Can you work these out from the model? Positions are in its coordinate system, mm. Face numbers are marked on the shaded views. A direction names the side the tool comes from. Coordinates: 2 decimals unless noted, no trailing zeros. Order: outer loops, then holes, each group sorted by start corner. A loop starts at its lowest first (then second) coordinate and runs counter-clockwise, first axis right, second up. Notation, with made-up numbers: (59.5, 45) -> (78.5, 45) arc R34 cw to (78.5, 77) -> close; hole circle Ø7 at (-32.5, 84). An arc over 180 degrees is marked (long way). Answer as a JSON object with one key per item and string values. Group by question number.
(1) I want a section at B-B, the plane y = 11.7. State how many separate pieces and enclosed holes the cut face has, plus the area to 3 significant figures.
(2) For pin 1 (1.2 mm diameter, centred on x = 8, y = 37, fed in from -Z); pin 2 (4 mm diameter, centred on x = 82.5, z = -12.5, fed in from -Y); pin 3 (0.8 mm diameter, centred on x = 130, y = 28.5, fed in from -Z), each with a flat end and sliding along its axis, tell me the tip position at first contact or that it passes through.
(3) I want a section at D-D, the plane y = 24. List the corners of the cut face in (x, z) for me, plus the area to 3 significant figures.
(4) I want a section at A-A, the plane z = -23. List the corners of the cut face in (x, y) for me, plus the area to 3 significant figures.
(5) I need wall thicknesses on line 1 (Y direction, x = 7.25, z = -13.25); line 2 (X direction, y = 37, z = -5); line 3 (Y direction, x = 129.75, z = -21). Which ranges of each line are inside material? Lowest first, please.
(6) If we mould it in two halves opening along X, with no side actions, what happens to the marked faces 3, 4, 5 and 6? For each: pulls with the +X half, pulls with the -X half, needs draft (parallel to the pull), parting line crosses it, or undercut.
(7) Which directions (+Z, -Z, +X, -X, +Y, -Y) give clear straight access to the entire face, cutting with the end or side of a thin tool? Please do the marked faces 1 and 2.
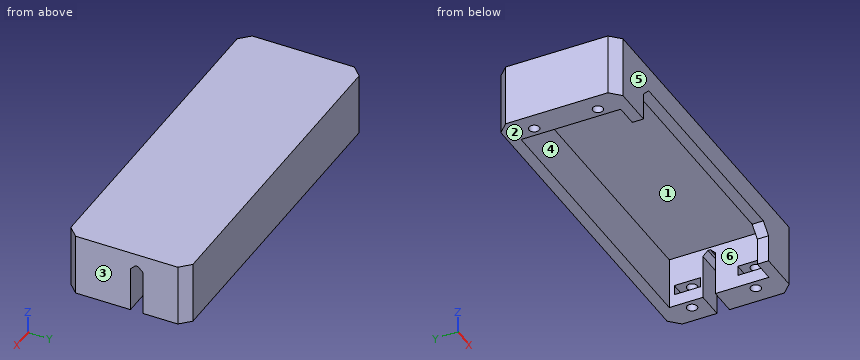
from build123d import *

# Parameters (mm, degrees)
SKETCH_W        = 137
SKETCH_H        = 49
SKETCH_R        = 2.05
SKETCH_W_2      = 115
SKETCH_H_2      = 40
PAD_DEPTH       = 25
CHAMFER_SIZE    = 4
SKETCH004_W     = 129
SKETCH004_H     = 41
PAD001_DEPTH    = 4
SKETCH003_W     = 7.55
SKETCH003_H     = 10.5
POCKET_DEPTH    = 4
POCKET001_DEPTH = 5.01
SKETCH005_W     = 22.132821
SKETCH005_H     = 5
POCKET002_DEPTH = 15
CHAMFER001_SIZE = 2


with BuildPart() as part:
    # Sketch → Pad (new body)
    with BuildSketch(Plane.XY):
        with Locations((68.5, 24.5)):
            Rectangle(SKETCH_W, SKETCH_H)
        with Locations((7.25, 11.7)):
            Circle(SKETCH_R, mode=Mode.SUBTRACT)
        with Locations((129.75, 11.7)):
            Circle(SKETCH_R, mode=Mode.SUBTRACT)
        with Locations((7.25, 37.3)):
            Circle(SKETCH_R, mode=Mode.SUBTRACT)
        with Locations((129.75, 37.3)):
            Circle(SKETCH_R, mode=Mode.SUBTRACT)
        with Locations((68.5, 24.5)):
            Rectangle(SKETCH_W_2, SKETCH_H_2, mode=Mode.SUBTRACT)
    extrude(amount=-PAD_DEPTH)

    # Chamfer
    chamfer_edges = [part.edges().sort_by_distance(p)[0] for p in [
        (137, 49, -12.5),
        (137, 0, -12.5),
        (0, 49, -12.5),
        (0, 0, -12.5),
    ]]
    chamfer(chamfer_edges, length=CHAMFER_SIZE)

    # Sketch004 → Pad001 (join)
    with BuildSketch(Plane.XY):
        with Locations((68.5, 24.5)):
            Rectangle(SKETCH004_W, SKETCH004_H)
    extrude(amount=-PAD001_DEPTH)

    # Sketch003 (on DatumPlane) → Pocket (cut)
    with BuildSketch(Plane.XY.offset(-20)):
        with Locations((7.25, 11.75)):
            Rectangle(SKETCH003_W, SKETCH003_H)
        with Locations((7.25, 37.25)):
            Rectangle(SKETCH003_W, SKETCH003_H)
        with Locations((129.75, 37.25)):
            Rectangle(SKETCH003_W, SKETCH003_H)
        with Locations((129.75, 11.75)):
            Rectangle(SKETCH003_W, SKETCH003_H)
    extrude(amount=POCKET_DEPTH, mode=Mode.SUBTRACT)

    # Sketch002 → Pocket001 (cut)
    with BuildSketch(Plane.XZ):
        Polygon((113, -10), (24, -10), (20, -14), (20, -147.795874), (117, -147.795874), (117, -14), align=None)
    extrude(amount=-POCKET001_DEPTH, mode=Mode.SUBTRACT)

    # Sketch005 (on DatumPlane) → Pocket002 (cut, symmetric)
    with BuildSketch(Plane.XY.offset(-20)):
        with Locations((131.19064, 28.5)):
            Rectangle(SKETCH005_W, SKETCH005_H)
    extrude(amount=POCKET002_DEPTH, both=True, mode=Mode.SUBTRACT)

    # Chamfer001
    chamfer001_edges = [part.edges().sort_by_distance(p)[0] for p in [
        (131.5, 26, -5),
        (131.5, 31, -5),
    ]]
    chamfer(chamfer001_edges, length=CHAMFER001_SIZE)


solid = part.part
Computed values:
{
 "1": {"separate pieces": "3", "enclosed holes": "0", "area": "810 mm2"},
 "2": {"pin 1": "stops at z = -4", "pin 2": "stops at y = 44.5", "pin 3": "stops at z = -5"},
 "3": {"outline": "(0, -25) -> (11, -25) -> (11, -4) -> (126, -4) -> (126, -25) -> (137, -25) -> (137, 0) -> (0, 0) -> close", "area": "1,010 mm2"},
 "4": {"outline": "(0, 4) -> (4, 0) -> (20, 0) -> (20, 4.5) -> (11, 4.5) -> (11, 44.5) -> (126, 44.5) -> (126, 31) -> (137, 31) -> (137, 45) -> (133, 49) -> (4, 49) -> (0, 45) -> close; (117, 0) -> (133, 0) -> (137, 4) -> (137, 26) -> (126, 26) -> (126, 4.5) -> (117, 4.5) -> close; hole circle Ø4.1 at (7.25, 11.7); hole circle Ø4.1 at (7.25, 37.3); hole circle Ø4.1 at (129.75, 11.7); hole circle Ø4.1 at (129.75, 37.3)", "area": "1,540 mm2"},
 "5": {"line 1": "y = 0 to 9.65, 13.75 to 35.25, 39.35 to 49", "line 2": "x = 0 to 5.22, 9.28 to 11, 126 to 127.72, 131.78 to 137", "line 3": "y = 0 to 9.65, 13.75 to 26, 31 to 35.25, 39.35 to 49"},
 "6": {"face 3": "pulls with the +X half", "face 4": "undercut", "face 5": "needs draft", "face 6": "undercut"},
 "7": {"face 1": "-Z", "face 2": "-Z, +X, -X, +Y, -Y"}
}
